For this review, use the dimensioned drawing (mm, ordinates from the lowest corner) and the shaded views. A direction names the side the tool comes from. Coordinates: 2 decimals unless noted, no trailing zeros. Loops run counter-clockwise (first coordinate to the right, second up) from the corner with the lowest first, then second, coordinate; pieces in that order, holes last. Notation, with made-up numbers: (44, 43.5) -> (101, 43.5) arc R23 ccw to (101, 75.5) -> close; hole circle Ø2 at (19.5, -19). An arc over 180 degrees is marked (long way). One line per question, with ' | ' between items. Start each with the question number.
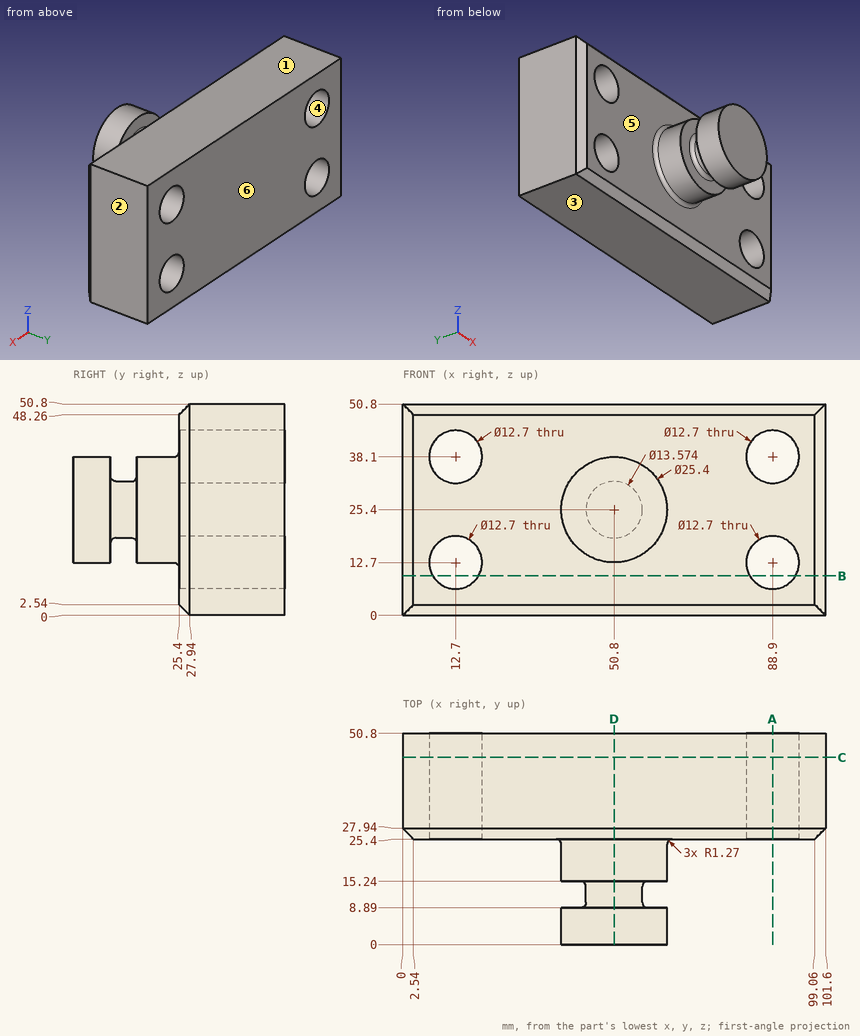
1) Machinability: for the marked faces 5 and 6, which of the approach directions +Z, -Z, +X, -X, +Y, -Y give a long, thin tool a straight path to every point of the face, cutting with its end or side? Answer none if there is none.
2) Consider section C-C, the plane y = 45. Write out the cut boundary in (x, z).
3) Insertion check: pin 1 Ø10 at (y, z) = (20, 10.5) entering from -X (1 decimal); pin 2 Ø7.5 at (x, z) = (12.7, 38.1) entering from -Y; pin 3 Ø14.5 at (x, z) = (12.7, 12.7) entering from -Y; pin 4 Ø7.5 at (x, z) = (51.5, 27) entering from -Y. Each pin has a flat end and moves straight along its axis. Give the tip position at first contact, or say it passes through.
4) Consider section D-D, the plane x = 50.8. Write out the cut boundary in (y, z).
5) Consider section A-A, the plane x = 88.9. Write out the cut boundary in (y, z).
6) Mouldability with a two-part tool opening along Z and no side actions: class the marked faces 1, 2, 3 and 4 as +Z half, -Z half, draft (parallel to the pull), parting line (faces both ways), or undercut.
7) Consider section B-B, the plane z = 9.5. Write out the cut boundary in (x, y) (1 decimal).
8) Wall thickness on L1, parallel to Z at x = 88, y = 40 (1 decimal); L2, parallel to X at y = 40, z = 12; L3, parallel to Z at x = 86, y = 38: over which ranges is each line inside the solid? List them lowest first.
Filled sheet:
1) face 5: -Y | face 6: +Z, -Z, +X, -X, +Y
2) outline: (0, 0) -> (101.6, 0) -> (101.6, 50.8) -> (0, 50.8) -> close; hole circle Ø12.7 at (12.7, 12.7); hole circle Ø12.7 at (12.7, 38.1); hole circle Ø12.7 at (88.9, 12.7); hole circle Ø12.7 at (88.9, 38.1)
3) pin 1: x = 42.8 | pin 2: through | pin 3: y = 25.4 | pin 4: y = 0
4) outline: (0, 12.7) -> (8.89, 12.7) -> (8.89, 17.34) arc R1.27 cw to (10.16, 18.61) -> (13.97, 18.61) arc R1.27 cw to (15.24, 17.34) -> (15.24, 12.7) -> (24.13, 12.7) arc R1.27 cw to (25.4, 11.43) -> (25.4, 2.54) -> (27.94, 0) -> (50.8, 0) -> (50.8, 50.8) -> (27.94, 50.8) -> (25.4, 48.26) -> (25.4, 39.37) arc R1.27 cw to (24.13, 38.1) -> (15.24, 38.1) -> (15.24, 33.46) arc R1.27 cw to (13.97, 32.19) -> (10.16, 32.19) arc R1.27 cw to (8.89, 33.46) -> (8.89, 38.1) -> (0, 38.1) -> close
5) outline: (25.4, 2.54) -> (27.94, 0) -> (50.8, 0) -> (50.8, 6.35) -> (25.4, 6.35) -> close; (25.4, 19.05) -> (50.8, 19.05) -> (50.8, 31.75) -> (25.4, 31.75) -> close; (25.4, 44.45) -> (50.8, 44.45) -> (50.8, 50.8) -> (27.94, 50.8) -> (25.4, 48.26) -> close
6) face 1: +Z half | face 2: draft | face 3: -Z half | face 4: undercut
7) outline: (0, 27.9) -> (2.5, 25.4) -> (7.2, 25.4) -> (7.2, 50.8) -> (0, 50.8) -> close; (18.2, 25.4) -> (83.4, 25.4) -> (83.4, 50.8) -> (18.2, 50.8) -> close; (94.4, 25.4) -> (99.1, 25.4) -> (101.6, 27.9) -> (101.6, 50.8) -> (94.4, 50.8) -> close
8) L1: 0 to 6.4, 19 to 31.8, 44.4 to 50.8 | L2: 0 to 6.39, 19.01 to 82.59, 95.21 to 101.6 | L3: 0 to 7.05, 18.35 to 32.45, 43.75 to 50.8
